from build123d import *

# Parameters (mm, degrees)
SKETCH1_W                   = 11
SKETCH1_H                   = 20
BASE_DEPTH                  = 4
SKETCH1_3_W                 = 11
SKETCH1_3_H                 = 8.089952371
SKETCH1_3_W_2               = 6.1
SKETCH1_3_H_2               = 2.8
VERTICALPIECE_DEPTH         = 13
FILLETCORNER_SIZE           = 3
FILLETCORNER_SIZE_2         = 5
F_3_2_3_2_HORIZONTAL_HOLE_D = 3.2
F_3_2_3_2_VERTICAL_HOLE_D   = 3.2
SKETCH1_4_W                 = 6.1
SKETCH1_4_H                 = 2.8
NUTSLOT_DEPTH               = 4.8
FILLET2_R                   = 2


with BuildPart() as part:
    # Sketch1 → Base (new body)
    with BuildSketch(Plane(origin=(0, 0, 0), x_dir=(1, 0, 0), z_dir=(0, 1, 0))):
        with Locations((0, 10)):
            Rectangle(SKETCH1_W, SKETCH1_H)
    extrude(amount=BASE_DEPTH)

    # Sketch1<3> → VerticalPiece (add)
    with BuildSketch(Plane(origin=(0, 0, 0), x_dir=(1, 0, 0), z_dir=(0, 1, 0))):
        with Locations((0, 4.044976186)):
            Rectangle(SKETCH1_3_W, SKETCH1_3_H)
        with Locations((0, 5.4)):
            Rectangle(SKETCH1_3_W_2, SKETCH1_3_H_2, mode=Mode.SUBTRACT)
    extrude(amount=VERTICALPIECE_DEPTH)

    # FilletCorner
    # an asymmetric fillet: 5, 3 mm, written as the material it adds along each edge
    with BuildSketch(Plane(origin=(-5.5, 4, -8.089952371), x_dir=(0, 0, -1), z_dir=(1, 0, 0))) as filletcorner_piece_1:
        with BuildLine():
            Bezier((FILLETCORNER_SIZE, 0), (0, 0), (0, FILLETCORNER_SIZE_2), weights=[1, 0.707106781, 1])
            Line((0, FILLETCORNER_SIZE_2), (0, 0))
            Line((0, 0), (FILLETCORNER_SIZE, 0))
        make_face()
    extrude(amount=11)

    # Ø3.2 (3.2) Horizontal Hole (through all)
    with Locations(Plane(origin=(0, 0, 0), x_dir=(-1, 0, 0), z_dir=(0, -1, 0))):
        with Locations((0, 15)):
            Hole(F_3_2_3_2_HORIZONTAL_HOLE_D / 2)

    # Ø3.2 (3.2) Vertical Hole (through all)
    with Locations(Plane.XY):
        with Locations((0, 8)):
            Hole(F_3_2_3_2_VERTICAL_HOLE_D / 2)

    # Sketch1<4> → NutSlot (add)
    with BuildSketch(Plane(origin=(0, 0, 0), x_dir=(1, 0, 0), z_dir=(0, 1, 0))):
        with Locations((0, 5.4)):
            Rectangle(SKETCH1_4_W, SKETCH1_4_H)
    extrude(amount=NUTSLOT_DEPTH)

    # Fillet2
    fillet2_edges = [part.edges().sort_by_distance(p)[0] for p in [
        (5.5, 2, -20),
        (-5.5, 2, -20),
        (-5.5, 13, -4.044976185),
        (5.5, 13, -4.044976185),
    ]]
    fillet(fillet2_edges, radius=FILLET2_R)


solid = part.part
Geometry check sheet. Reference: the model listing, model coordinates, mm. A direction names the side the tool comes from. Coordinates: 2 decimals unless noted, no trailing zeros. Order: outer loops, then holes, each group sorted by start corner. A loop starts at its lowest first (then second) coordinate and runs counter-clockwise, first axis right, second up. Notation, with made-up numbers: (17, 18) -> (65, 18) arc R18 ccw to (65, 40) -> close; hole circle Ø7 at (46, 43.5). An arc over 180 degrees is marked (long way). Use a Markdown table: item, result. Add a question column.
1. Mould release check, pull along X, two halves, no side actions. Record for faces 1 (the face through (-5.5, 4, -7)), 2 (the face through (0, 0, -10)), 3 (the face through (0, 10, -6.8)): pulls with the +X half, pulls with the -X half, needs draft (parallel to the pull), parting line crosses it, or undercut.
2. Cross-section at D-D (x = 1). Give the number of separate pieces and of enclosed holes in the cut face, and give its area (3 significant figures).
3. Set-up check for faces 4 (the face through (0, 11, -8.09)), 5 (the face through (-0.208, 2.028, -16.586)), 6 (the face through (0, 4.8, -5)): record each of +Z, -Z, +X, -X, +Y, -Y from which the full face is reachable in a straight line by a thin tool's end or side.
4. Cross-section at A-A (z = -15). Enter the section's corners in (x, y).
5. Go/stop test with flat-tipped pins: pin 1 Ø2 at (x, y) = (0.5, 11) entering from -Z; pin 2 Ø1.4 at (x, z) = (-1, -6) entering from +Y; pin 3 Ø4.5 at (x, z) = (0, -17) entering from +Y. Record where each tip stops, or that it passes through.
6. Cross-section at B-B (y = 3.75). Enter the section's corners in (x, z).
7. Cross-section at C-C (z = -1). Enter the section's corners in (x, y).
8. Material ranges on L1, parallel to Z at x = 0, y = 1.05; L2, parallel to Z at x = -2.5, y = 12.5; L3, parallel to Y at x = 0, z = -2.95, recorded low to high.
Filled sheet:
| question | item | result |
|---|---|---|
| 1 | face 1 | pulls with the -X half |
| 1 | face 2 | needs draft |
| 1 | face 3 | undercut |
| 2 | separate pieces | 4 |
| 2 | enclosed holes | 0 |
| 2 | area | 110 mm2 |
| 3 | face 4 | -Z, +X, -X, +Y |
| 3 | face 5 | +Y, -Y |
| 3 | face 6 | +Y |
| 4 | outline | (-5.5, 0) -> (-1.6, 0) -> (-1.6, 4) -> (-5.5, 4) -> close; (1.6, 0) -> (5.5, 0) -> (5.5, 4) -> (1.6, 4) -> close |
| 5 | pin 1 | z = -8.09 |
| 5 | pin 2 | y = 4.8 |
| 5 | pin 3 | y = 4 |
| 6 | outline | (-5.5, -18) arc R2 ccw to (-3.5, -20) -> (3.5, -20) arc R2 ccw to (5.5, -18) -> (5.5, 0) -> (-5.5, 0) -> close; hole circle Ø3.2 at (0, -15) |
| 7 | outline | (-5.5, 0) -> (5.5, 0) -> (5.5, 11) arc R2 ccw to (3.5, 13) -> (-3.5, 13) arc R2 ccw to (-5.5, 11) -> close; hole circle Ø3.2 at (0, 8) |
| 8 | L1 | -20 to -16.6, -13.4 to 0 |
| 8 | L2 | -8.09 to -6.8, -4 to 0 |
| 8 | L3 | 0 to 6.4, 9.6 to 13 |
